from build123d import *

# Parameters (mm, degrees)
CROQUIS1_R              = 150
CROQUIS1_R_2            = 3.25
SALIENTE_EXTRUIR1_DEPTH = 2
CROQUIS2_W              = 26
CROQUIS2_H              = 26
CORTAR_EXTRUIR1_DEPTH   = 213.141462237


with BuildPart() as part:
    # Croquis1 → Saliente-Extruir1 (new body)
    with BuildSketch(Plane.XY):
        Circle(CROQUIS1_R)
        with Locations((140, 0)):
            Circle(CROQUIS1_R_2, mode=Mode.SUBTRACT)
        with Locations((0, -140)):
            Circle(CROQUIS1_R_2, mode=Mode.SUBTRACT)
        with Locations((-140, 0)):
            Circle(CROQUIS1_R_2, mode=Mode.SUBTRACT)
        with Locations((0, 140)):
            Circle(CROQUIS1_R_2, mode=Mode.SUBTRACT)
    extrude(amount=SALIENTE_EXTRUIR1_DEPTH)

    # Croquis2 → Cortar-Extruir1 (cut, through all)
    with BuildSketch(Plane.XY.offset(2)):
        Rectangle(CROQUIS2_W, CROQUIS2_H)
    extrude(amount=-CORTAR_EXTRUIR1_DEPTH, mode=Mode.SUBTRACT)


solid = part.part
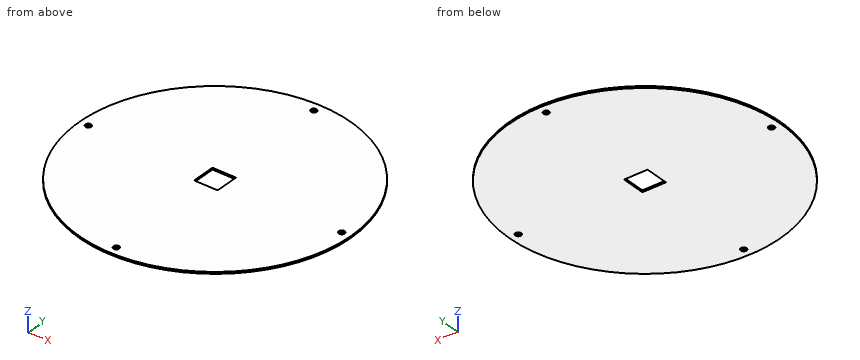
The listing builds one solid part. Answer for the finished solid, in the listing's coordinates (mm). Give positions to 0.01 mm unless a question says otherwise; leave off trailing zeros. Write each loop counter-clockwise with the first axis right and the second up, starting at its lowest first coordinate (ties: lowest second). Pieces come first, ordered by that corner, then holes.
1) Find the intervals of material crossed by L1, parallel to Y at x = 0, z = 0.9; L2, parallel to X at y = -1.5, z = 1.4; L3, parallel to X at y = -9, z = 0.1, in increasing order.
2) Given P1, Ø5, axis at x = -140, y = 0, coming from the +Z side, flat-ended and moving along its own axis, determine where the tip first touches the part or whether it passes through.
3) Section A-A (z = 0.9) is taken. Write down the section's boundary in (x, y), and give its area (3 significant figures).
4) Section B-B (x = -122.5) is taken. Write down the section's boundary in (y, z), and give its area (3 significant figures).
5) Section C-C (y = 119) is taken. Write down the section's boundary in (x, z).
Response:
1. L1: y = -150 to -143.25, -136.75 to -13, 13 to 136.75, 143.25 to 150
1. L2: x = -149.99 to -142.88, -137.12 to -13, 13 to 137.12, 142.88 to 149.99
1. L3: x = -149.73 to -13, 13 to 149.73
2. P1: passes through
3. outline: circle Ø300 at (0, 0); hole circle Ø6.5 at (-140, 0); hole (-13, -13) - (13, -13) - (13, 13) - (-13, 13) - close; hole circle Ø6.5 at (0, -140); hole circle Ø6.5 at (0, 140); hole circle Ø6.5 at (140, 0)
3. area: 69,900 mm2
4. outline: (-86.57, 0) - (86.57, 0) - (86.57, 2) - (-86.57, 2) - close
4. area: 346 mm2
5. outline: (-91.32, 0) - (91.32, 0) - (91.32, 2) - (-91.32, 2) - close
